Here's how the part is built. I have some questions about the finished solid (model axes, mm). Face numbers are marked on the shaded views. A direction names the side the tool comes from. Coordinates: 2 decimals unless noted, no trailing zeros. Write each loop counter-clockwise with the first axis right and the second up, starting at its lowest first coordinate (ties: lowest second). Pieces come first, ordered by that corner, then holes.
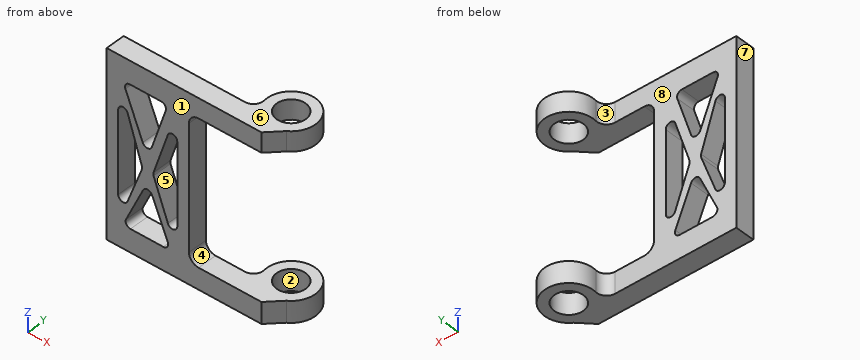
```python
from build123d import *

# Parameters (mm, degrees)
F0_R      = 3
F1_DEPTH  = 38
F3_W      = 47.0337605621
F3_H      = 38
F4_DEPTH  = 2
F6_DEPTH  = 38
F7_DEPTH  = 12.5
F9_DEPTH  = 25
F10_R     = 1
F11_W     = 18.2646340574
F11_H     = 47.5416160189
F12_DEPTH = 25


with BuildPart() as f1:
    # F0 (on Top) → F1 (new body)
    with BuildSketch(Plane.XY):
        with BuildLine():
            Line((-30.015476048, 0), (17.0182845141, 0))
            ThreePointArc((17.0182845141, 0), (20.2915528676, 8.7796447301), (12.069567921, 4.2857142857))
            ThreePointArc((12.069567921, 4.2857142857), (11.6019391758, 2.6906926586), (10.0900812838, 2))
            Line((10.0900812838, 2), (-30.015476048, 2))
            Line((-30.015476048, 2), (-30.015476048, 0))
        make_face()
        with Locations((17.0182845141, 5)):
            Circle(F0_R, mode=Mode.SUBTRACT)
    extrude(amount=F1_DEPTH)

    # F3 (on face) → F4 (join)
    with BuildSketch(Plane.XZ):
        with Locations((-6.498595767, 19)):
            Rectangle(F3_W, F3_H)
    extrude(amount=F4_DEPTH)

    # F5 (on face) → F6 (join)
    with BuildSketch(Plane(origin=(0, 0, 0), x_dir=(1, 0, 0), z_dir=(0, 0, -1))):
        with BuildLine():
            Line((19.7223976995, -0.7943167166), (17.0182845141, 2))
            Line((17.0182845141, 2), (17.0182845141, 0))
            ThreePointArc((17.0182845141, 0), (18.4274657627, -0.2026873973), (19.7223976995, -0.7943167166))
        make_face()
    extrude(amount=-F6_DEPTH)

    # F2 (on face) → F7 (cut, symmetric)
    with BuildSketch(Plane.XZ):
        with BuildLine():
            Line((-16.9817154859, 33.5), (-30.015476048, 33.5))
            Line((-30.015476048, 33.5), (-30.015476048, 4.5))
            Line((-30.015476048, 4.5), (-16.9817154859, 4.5))
            ThreePointArc((-16.9817154859, 4.5), (-15.5675019236, 5.0857864376), (-14.9817154859, 6.5))
            Line((-14.9817154859, 6.5), (-14.9817154859, 31.5))
            ThreePointArc((-14.9817154859, 31.5), (-15.5675019236, 32.9142135624), (-16.9817154859, 33.5))
        make_face()
        with BuildLine():
            Line((38.1005785107, 4.3682365306), (38.1005785107, 33.9556627348))
            Line((38.1005785107, 33.9556627348), (4.0182845141, 33.9556627348))
            ThreePointArc((4.0182845141, 33.9556627348), (2.6040709517, 33.3698762972), (2.0182845141, 31.9556627348))
            Line((2.0182845141, 31.9556627348), (2.0182845141, 6.3682365306))
            ThreePointArc((2.0182845141, 6.3682365306), (2.6040709517, 4.9540229682), (4.0182845141, 4.3682365306))
            Line((4.0182845141, 4.3682365306), (38.1005785107, 4.3682365306))
        make_face()
    extrude(amount=F7_DEPTH, both=True, mode=Mode.SUBTRACT)

    # F8 (on face) → F9 (cut)
    with BuildSketch(Plane.XZ.offset(2)):
        Polygon((-7.5863441452, 18.0459246039), (-12.6038566232, 33.2977212965), (-12.6038566232, 4.6920240857), align=None)
        Polygon((-0.3933349107, 33.2977212965), (-5.4108473887, 18.0459246039), (-0.3933349107, 4.6920240857), align=None)
        Polygon((-2.3342688624, 33.2977212965), (-11.6795975956, 33.2977212965), (-6.498595767, 20.6393636763), align=None)
        Polygon((-1.7651436112, 4.6920240857), (-6.498595767, 15.827909112), (-11.6411998855, 4.6920240857), align=None)
    extrude(amount=-F9_DEPTH, mode=Mode.SUBTRACT)

    # F10
    f10_edges = [f1.edges().sort_by_distance(p)[0] for p in [
        (-11.679598, 0, 33.297721),
        (-2.334269, 0, 33.297721),
        (-12.603857, 0, 33.297721),
        (-12.603857, 0, 4.692024),
        (-7.586344, 0, 18.045925),
        (-6.498596, 0, 20.639364),
        (-0.393335, 0, 33.297721),
        (-5.410847, 0, 18.045925),
        (-0.393335, 0, 4.692024),
        (-6.498596, 0, 15.827909),
        (-1.765144, 0, 4.692024),
        (-11.6412, 0, 4.692024),
    ]]
    fillet(f10_edges, radius=F10_R)

    # F11 (on face) → F12 (cut)
    with BuildSketch(Plane.XZ.offset(2)):
        with Locations((-24.1140325146, 18.5290810186)):
            Rectangle(F11_W, F11_H)
    extrude(amount=-F12_DEPTH, mode=Mode.SUBTRACT)


solid = f1.part
```
1) Imagine slicing it at A-A on y = 5. Please give me the cut outline in (x, z).
Values follow:
outline: (12.02, 0) - (14.02, 0) - (14.02, 4.37) - (12.02, 4.37) - close; (12.02, 33.96) - (14.02, 33.96) - (14.02, 38) - (12.02, 38) - close; (20.02, 0) - (22.02, 0) - (22.02, 4.37) - (20.02, 4.37) - close; (20.02, 33.96) - (22.02, 33.96) - (22.02, 38) - (20.02, 38) - close
2) Will these pins go through, and if not, where does the flat tip stop? pin 1 (5 mm diameter, centred on x = 14, y = 4, fed in from -Z); pin 2 (2 mm diameter, centred on x = 11, y = 7.5, fed in from +Z); pin 3 (3 mm diameter, centred on y = -1, z = 14, fed in from +X).
Values follow:
pin 1: stops at z = 0
pin 2: passes through
pin 3: stops at x = 2.02
3) Imagine slicing it at C-C on z = 32.5. Please give me the cut outline in (x, y), then the cut area to 3 significant figures.
Values follow:
outline: (-14.98, -2) - (-11.17, -2) - (-11.17, 2) - (-14.98, 2) - close; (-2.74, -2) - (2.09, -2) - (2.09, 2) - (-2.74, 2) - close
area: 34.6 mm2
4) Imagine slicing it at B-B on x = 4.5. Please give me the cut outline in (y, z).
Values follow:
outline: (-2, 0) - (2, 0) - (2, 4.37) - (-2, 4.37) - close; (-2, 33.96) - (2, 33.96) - (2, 38) - (-2, 38) - close
5) We'd pull the mould along X, two halves only. Please class the marked faces 1, 2 and 3: pulls with the +X half, pulls with the -X half, needs draft (parallel to the pull), parting line crosses it, or undercut.
Values follow:
face 1: needs draft
face 2: undercut
face 3: pulls with the -X half
6) Imagine slicing it at D-D on x = -6.5. Please give me the cut outline in (y, z), then the cut area to 3 significant figures.
Values follow:
outline: (-2, 0) - (2, 0) - (2, 4.69) - (-2, 4.69) - close; (-2, 14.36) - (2, 14.36) - (2, 22.53) - (-2, 22.53) - close; (-2, 33.3) - (2, 33.3) - (2, 38) - (-2, 38) - close
area: 70.3 mm2
7) On a 3-axis mill with a long thin cutter (end or side, diameter ignored), from which of +Z, -Z, +X, -X, +Y, -Y can I reach the whole of each face in a straight line? I mean the marked faces 4, 5, 6, 7 and 8. Say none if no direction works.
Values follow:
face 4: +X, +Y, -Y
face 5: +Y, -Y
face 6: +Z, +X, -X, +Y, -Y
face 7: +Z, -Z, -X, +Y, -Y
face 8: +Z, -Z, -X, +Y
8) I need wall thicknesses on probe 1 along Z at (x, y) = (18, 9.75); probe 2 along X at (y, z) = (5, 0.9); probe 3 along Y at (x, z) = (-12.5, 9). Which ranges of each line are inside material? Lowest first, please.
Values follow:
probe 1: z = 0 to 4.37, 33.96 to 38
probe 2: x = 12.02 to 14.02, 20.02 to 22.02
probe 3: y = -2 to 2
